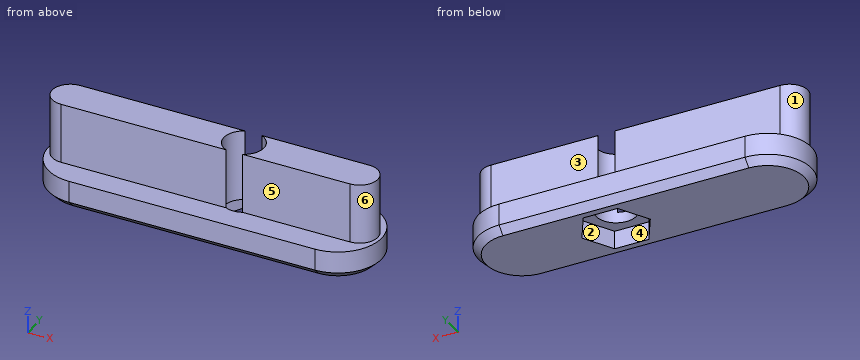
```python
from build123d import *

# Parameters (mm, degrees)
PAD_DEPTH       = 4
PAD001_DEPTH    = 8.3
SKETCH002_R     = 2.75
POCKET_DEPTH    = 12.301
POCKET001_DEPTH = 2.5
CHAMFER_SIZE    = 1


with BuildPart() as part:
    # Sketch → Pad (new body)
    with BuildSketch(Plane.XY):
        with BuildLine():
            ThreePointArc((-17, 6), (-23, 0), (-17, -6))
            Line((-17, -6), (17, -6))
            ThreePointArc((17, -6), (23, 0), (17, 6))
            Line((-17, 6), (17, 6))
        make_face()
    extrude(amount=PAD_DEPTH)

    # Sketch001 → Pad001 (new body)
    with BuildSketch(Plane.XY.offset(4)):
        with BuildLine():
            ThreePointArc((-20, 2.5), (-22.5, 0), (-20, -2.5))
            Line((-20, -2.5), (20, -2.5))
            ThreePointArc((20, -2.5), (22.5, 0), (20, 2.5))
            Line((-20, 2.5), (20, 2.5))
        make_face()
    extrude(amount=PAD001_DEPTH)

    # Sketch002 → Pocket (cut, through all)
    with BuildSketch(Plane.XY.offset(12.3)):
        with Locations((4, 0)):
            Circle(SKETCH002_R)
    extrude(amount=-POCKET_DEPTH, mode=Mode.SUBTRACT)

    # Sketch003 → Pocket001 (cut)
    with BuildSketch(Plane(origin=(0, 0, 0), x_dir=(1, 0, 0), z_dir=(0, 0, -1))):
        Polygon((8.734272, 0), (6.367136, 4.1), (1.632864, 4.1), (-0.734272, 0), (1.632864, -4.1), (6.367136, -4.1), align=None)
    extrude(amount=-POCKET001_DEPTH, mode=Mode.SUBTRACT)

    # Chamfer
    chamfer_edges = [part.edges().sort_by_distance(p)[0] for p in [
        (0, -6, 0),
    ]]
    chamfer(chamfer_edges, length=CHAMFER_SIZE)


solid = part.part
```
Input: part model. Units: mm. Frame: model coordinates. Face numbers are marked on the shaded views. A direction names the side the tool comes from. Coordinates: 2 decimals unless noted, no trailing zeros. Loops run counter-clockwise (first coordinate to the right, second up) from the corner with the lowest first, then second, coordinate; pieces in that order, holes last. Notation, with made-up numbers: M 80.5,61 L 88.5,61 A27 ccw 88.5,87 Z; hole C 76.25,-14.75 d2. An arc over 180 degrees is marked long. Use a Markdown table: item, result. Add a question column.
1) Pin query (flat end, axial travel): P1, Ø4.5, axis at x = 4, y = 0, coming from the +Z side; P2, Ø2.5, axis at x = -7, z = 8, coming from the -Y side; P3, Ø1.5, axis at y = 3, z = 9.5, coming from the -X side; P4, Ø1.5, axis at y = 1.5, z = 4, coming from the -X side. Return the tip coordinate at first contact, or that it passes through.
2) Line query: L1, parallel to X at y = 0, z = 6.5; L2, parallel to Z at x = -11, y = 4.25; L3, parallel to Y at x = -0.5, z = 10.25. Output: solid intervals per line, ascending. Write a range as from..to.
3) Section B-B, the plane x = 4. Return the cut outline in (y, z), plus the area to 4 significant figures.
4) Draft query along X for the marked faces 4, 5 and 6. Return one class per face: +X half, -X half, draft (parallel to the pull), parting line (faces both ways), or undercut.
5) Section C-C, the plane x = -11.5. Return the cut outline in (y, z), plus the area to 3 significant figures.
6) Section A-A, the plane z = 7. Return the cut outline in (x, y).
7) Set-up query: the marked faces 1, 2 and 3. Return all of +Z, -Z, +X, -X, +Y, -Y with unobstructed straight access to the full face (end or side cutting, diameter ignored); none if empty.
Answer below:
| question | item | result |
|---|---|---|
| 1 | P1 | through |
| 1 | P2 | y = -2.5 |
| 1 | P3 | x = -21.09 |
| 1 | P4 | x = -22.95 |
| 2 | L1 | -22.5..1.25, 6.75..22.5 |
| 2 | L2 | 0..4 |
| 2 | L3 | -2.5..2.5 |
| 3 | outline | M -6,1 L -5,0 L -4.1,0 L -4.1,2.5 L -2.75,2.5 L -2.75,4 L -6,4 Z; M 2.75,2.5 L 4.1,2.5 L 4.1,0 L 5,0 L 6,1 L 6,4 L 2.75,4 Z |
| 3 | area | 18.25 mm2 |
| 4 | face 4 | undercut |
| 4 | face 5 | draft |
| 4 | face 6 | +X half |
| 5 | outline | M -6,1 L -5,0 L 5,0 L 6,1 L 6,4 L 2.5,4 L 2.5,12.3 L -2.5,12.3 L -2.5,4 L -6,4 Z |
| 5 | area | 88.5 mm2 |
| 6 | outline | M -20,-2.5 L 2.85,-2.5 A2.75 cw 2.85,2.5 L -20,2.5 A2.5 ccw Z; M 5.15,-2.5 L 20,-2.5 A2.5 ccw 20,2.5 L 5.15,2.5 A2.75 cw Z |
| 7 | face 1 | +Z, -X |
| 7 | face 2 | -Z |
| 7 | face 3 | +Z, +X, -X, +Y |
